Part model, mm, in its own coordinate system. A direction names the side the tool comes from. Round coordinates to 2 decimals unless told otherwise and drop trailing zeros. Write each loop counter-clockwise with the first axis right and the second up, starting at its lowest first coordinate (ties: lowest second). Pieces come first, ordered by that corner, then holes.
from build123d import *

# Parameters (mm, degrees)
SKETCH1_R           = 4
BOSS_EXTRUDE1_DEPTH = 170
SKETCH16_W          = 6
SKETCH16_H          = 3


with BuildPart() as part:
    # Sketch1 → Boss-Extrude1 (new body)
    with BuildSketch(Plane(origin=(0, 0, 0), x_dir=(1, 0, 0), z_dir=(0, 1, 0))):
        with Locations(Location((0, 0, 0), (0, 0, 270))):
            Circle(SKETCH1_R)
    extrude(amount=BOSS_EXTRUDE1_DEPTH)

    # Sketch16 → Revolve1 (revolve)
    with BuildSketch(Plane.XY, mode=Mode.PRIVATE) as revolve1_sk:
        with Locations((3, 136.5)):
            Rectangle(SKETCH16_W, SKETCH16_H)
    revolve(revolve1_sk.sketch.rotate(Axis((0, 135, 0), (0, 1, 0)), 90), axis=Axis((0, 135, 0), (0, 1, 0)))


solid = part.part
Q1. Drop flat-ended pins along their axis: P1, Ø4, axis at y = 41.5, z = -2.5, coming from the +X side; P2, Ø2, axis at x = -0.5, y = 18, coming from the -Z side; P3, Ø6, axis at x = 1, z = 0.5, coming from the -Y side; P4, Ø4, axis at y = 103.5, z = -3, coming from the -X side. Give the stop position or say it passes through.
Q2. Wall check: line 1 (Y direction, x = -4.25, z = -2); line 2 (Z direction, x = 0, y = 124.5); line 3 (X direction, y = 116.5, z = -0.5). Give the ranges that are in metal, low to high.
Q3. Saw through at C-C, the plane y = 140.5. Write the cut outline in (x, z), and give its area (3 significant figures).
Q4. Saw through at B-B, the plane x = 0. Write the cut outline in (y, z), and give its area (3 significant figures).
Q5. Tool access for faces 1 (the flat face through (3.92, 138, -1.42)), 2 (the flat face through (0, 170, 0)), 3 (the cylindrical face through (-3.905, 66.555, -0.867)): list every direction of +Z, -Z, +X, -X, +Y, -Y with a clear straight run to the whole face (end or side of a thin tool).
Q6. Saw through at A-A, the plane z = 0. Write the cut outline in (x, y), and give its area (3 significant figures).
Computed:
1. P1: stops at x = 3.97
1. P2: stops at z = -4
1. P3: stops at y = 0
1. P4: stops at x = -3.87
2. line 1: y = 135 to 138
2. line 2: z = -4 to 4
2. line 3: x = -3.97 to 3.97
3. outline: circle Ø8 at (0, 0)
3. area: 50.3 mm2
4. outline: (0, -4) - (135, -4) - (135, -6) - (138, -6) - (138, -4) - (170, -4) - (170, 4) - (138, 4) - (138, 6) - (135, 6) - (135, 4) - (0, 4) - close
4. area: 1,370 mm2
5. face 1: +Y
5. face 2: +Z, -Z, +X, -X, +Y
5. face 3: -Y
6. outline: (-6, 135) - (-4, 135) - (-4, 0) - (4, 0) - (4, 135) - (6, 135) - (6, 138) - (4, 138) - (4, 170) - (-4, 170) - (-4, 138) - (-6, 138) - close
6. area: 1,370 mm2
